Can you work these out from the drawing? Everything is in mm from the part's minimum corner. Coordinates: 2 decimals unless noted, no trailing zeros. Write each loop counter-clockwise with the first axis right and the second up, starting at its lowest first coordinate (ties: lowest second). Pieces come first, ordered by that corner, then holes.
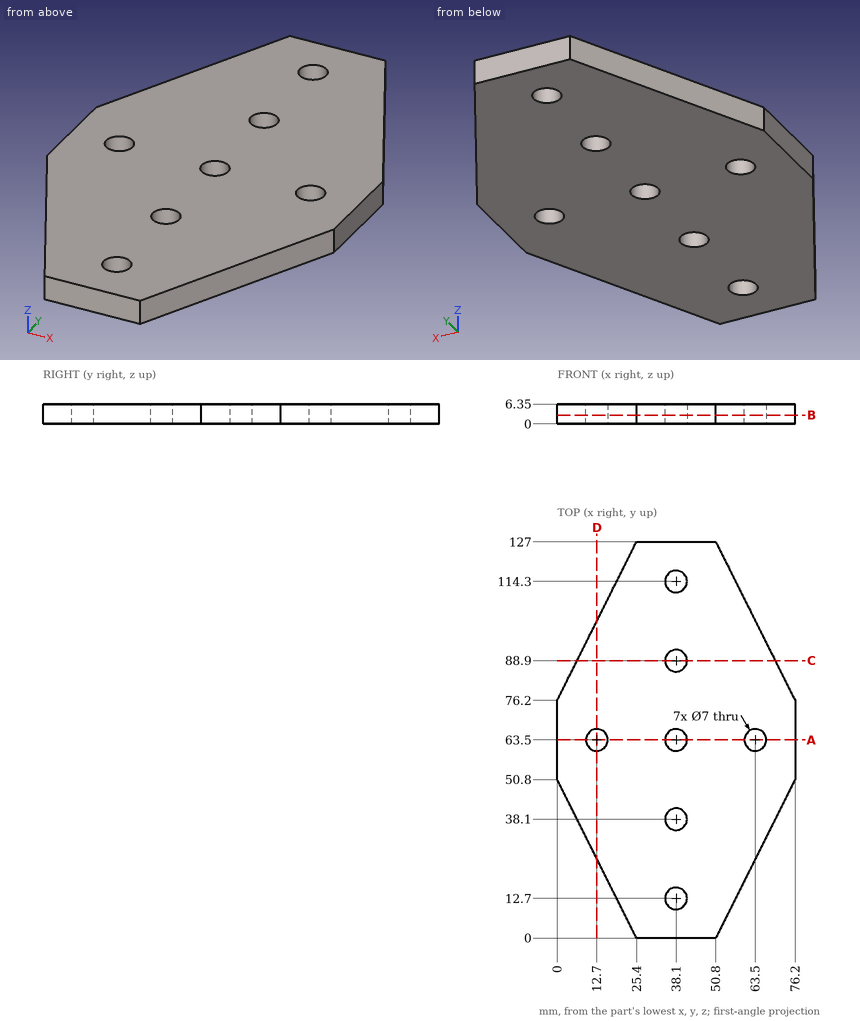
1. For pin 1 Ø1 at (y, z) = (47.5, 4.5) entering from +X; pin 2 Ø1.5 at (y, z) = (47, 5.5) entering from +X (3 decimals), each with a flat end and sliding along its axis, tell me the tip position at first contact or that it passes through.
2. I want a section at D-D (x = 12.7). List the corners of the cut face in (y, z) for me.
3. I want a section at C-C (y = 88.9). List the corners of the cut face in (x, z) for me.
4. I want a section at A-A (y = 63.5). List the corners of the cut face in (x, z) for me.
5. If I drill on line 1 (Y direction, x = 38.1, z = 5.25); line 2 (Y direction, x = 37, z = 2.5); line 3 (Y direction, x = 66.5, z = 2), over which ranges is the centre line in solid material (lowest first)?
6. I want a section at B-B (z = 2.75). List the corners of the cut face in (x, y) for me.
Response values:
1. pin 1: stops at x = 74.8
1. pin 2: stops at x = 74.675
2. outline: (25.4, 0) - (60, 0) - (60, 6.35) - (25.4, 6.35) - close; (67, 0) - (101.6, 0) - (101.6, 6.35) - (67, 6.35) - close
3. outline: (6.35, 0) - (34.6, 0) - (34.6, 6.35) - (6.35, 6.35) - close; (41.6, 0) - (69.85, 0) - (69.85, 6.35) - (41.6, 6.35) - close
4. outline: (0, 0) - (9.2, 0) - (9.2, 6.35) - (0, 6.35) - close; (16.2, 0) - (34.6, 0) - (34.6, 6.35) - (16.2, 6.35) - close; (41.6, 0) - (60, 0) - (60, 6.35) - (41.6, 6.35) - close; (67, 0) - (76.2, 0) - (76.2, 6.35) - (67, 6.35) - close
5. line 1: y = 0 to 9.2, 16.2 to 34.6, 41.6 to 60, 67 to 85.4, 92.4 to 110.8, 117.8 to 127
5. line 2: y = 0 to 9.38, 16.02 to 34.78, 41.42 to 60.18, 66.82 to 85.58, 92.22 to 110.98, 117.62 to 127
5. line 3: y = 31.4 to 61.7, 65.3 to 95.6
6. outline: (0, 50.8) - (25.4, 0) - (50.8, 0) - (76.2, 50.8) - (76.2, 76.2) - (50.8, 127) - (25.4, 127) - (0, 76.2) - close; hole circle Ø7 at (12.7, 63.5); hole circle Ø7 at (38.1, 12.7); hole circle Ø7 at (38.1, 38.1); hole circle Ø7 at (38.1, 63.5); hole circle Ø7 at (38.1, 88.9); hole circle Ø7 at (38.1, 114.3); hole circle Ø7 at (63.5, 63.5)
